The figure shows three views and two pictorial views of one solid part (mm, origin at its lowest corner). Answer the questions. A direction names the side the tool comes from. Give positions to 0.01 mm unless a question says otherwise; leave off trailing zeros. Order: outer loops, then holes, each group sorted by start corner. A loop starts at its lowest first (then second) coordinate and runs counter-clockwise, first axis right, second up. Notation, with made-up numbers: (12.5, 70.5) - (17.5, 70.5) arc R10 cw to (17.5, 83.5) - close; hole circle Ø2 at (33.25, 13). An arc over 180 degrees is marked (long way). Use a Markdown table: item, result. Add a question column.
1. A cutting plane is placed at D-D on y = 6.5. Determine the outline of the cut face in (x, z).
2. For a pull along X with two mould halves and no side action, classify the marked faces 3, 4 and 5 as released by +X, released by -X, zero draft, split by the parting line, or undercut.
3. Consider L1, parallel to Z at x = 42.5, y = 6; L2, parallel to Z at x = 53.5, y = 9; L3, parallel to Y at x = 4.5, z = 40. Determine where each line is inside the solid, lowest interval first.
4. A cutting plane is placed at B-B on y = 1.5. Determine the outline of the cut face in (x, z), and give its area (3 significant figures).
5. A cutting plane is placed at A-A on x = 42.5. Determine the outline of the cut face in (y, z), and give its area (3 significant figures).
6. Which of the six approach directions +Z, -Z, +X, -X, +Y, -Y give full straight-line access (tool end or side, diameter ignored) to the marked faces 1 and 2?
7. Flat-ended cylindrical pins translate along their axes: P1, Ø9.5, axis at x = 42, z = 34, coming from the +Y side; P2, Ø2, axis at y = 5.5, z = 36.5, coming from the -X side; P3, Ø3, axis at x = 61, z = 16, coming from the -Y side; P4, Ø1, axis at y = 8, z = 15, coming from the +X side. Find the tip coordinate at first contact, or state that the pin passes through.
8. A cutting plane is placed at C-C on x = 20.5. Determine the outline of the cut face in (y, z).
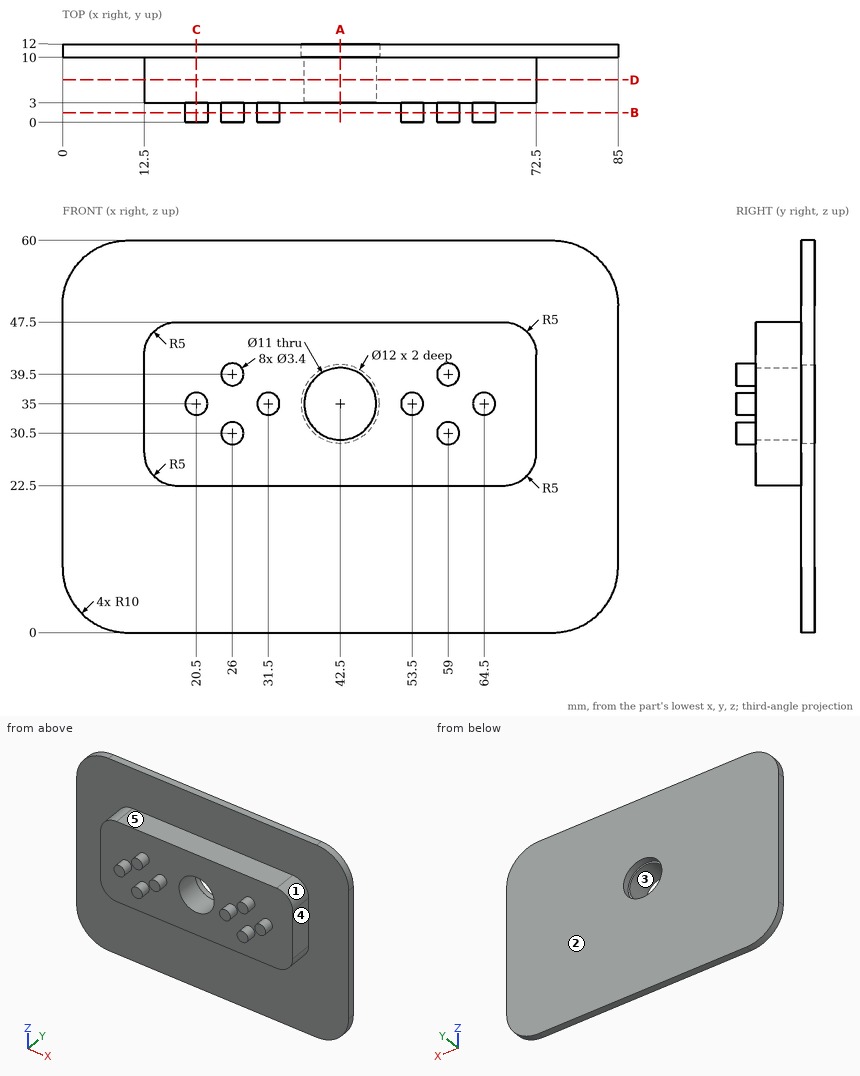
Output values:
| question | item | result |
|---|---|---|
| 1 | outline | (12.5, 27.5) arc R5 ccw to (17.5, 22.5) - (67.5, 22.5) arc R5 ccw to (72.5, 27.5) - (72.5, 42.5) arc R5 ccw to (67.5, 47.5) - (17.5, 47.5) arc R5 ccw to (12.5, 42.5) - close; hole circle Ø11 at (42.5, 35) |
| 2 | face 3 | undercut |
| 2 | face 4 | released by +X |
| 2 | face 5 | zero draft |
| 3 | L1 | 22.5 to 29.5, 40.5 to 47.5 |
| 3 | L2 | 22.5 to 47.5 |
| 3 | L3 | 10 to 12 |
| 4 | outline | circle Ø3.4 at (20.5, 35); circle Ø3.4 at (26, 30.5); circle Ø3.4 at (26, 39.5); circle Ø3.4 at (31.5, 35); circle Ø3.4 at (53.5, 35); circle Ø3.4 at (59, 30.5); circle Ø3.4 at (59, 39.5); circle Ø3.4 at (64.5, 35) |
| 4 | area | 72.6 mm² |
| 5 | outline | (3, 22.5) - (10, 22.5) - (10, 0) - (12, 0) - (12, 29) - (10, 29) - (10, 29.5) - (3, 29.5) - close; (3, 40.5) - (10, 40.5) - (10, 41) - (12, 41) - (12, 60) - (10, 60) - (10, 47.5) - (3, 47.5) - close |
| 5 | area | 194 mm² |
| 6 | face 1 | +Z, +X, -Y |
| 6 | face 2 | +Z, -Z, +X, -X, +Y |
| 7 | P1 | y = 10 |
| 7 | P2 | x = 12.5 |
| 7 | P3 | y = 10 |
| 7 | P4 | through |
| 8 | outline | (0, 33.3) - (3, 33.3) - (3, 22.5) - (10, 22.5) - (10, 0) - (12, 0) - (12, 60) - (10, 60) - (10, 47.5) - (3, 47.5) - (3, 36.7) - (0, 36.7) - close |
